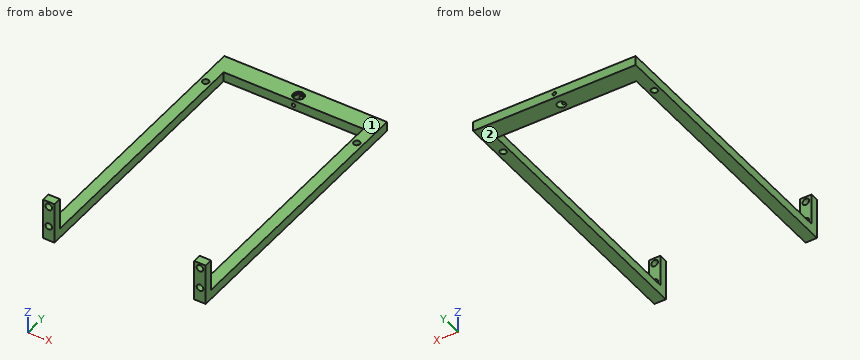
from build123d import *

# Parameters (mm, degrees)
SKETCH1_W           = 99.5426
SKETCH1_H           = 5.842
BOSS_EXTRUDE1_DEPTH = 170.18
SKETCH2_W           = 85.471
SKETCH2_H           = 158.8
CUT_EXTRUDE1_DEPTH  = 232.802638094
SKETCH3_W           = 7.0358
SKETCH3_H           = 5.08
BOSS_EXTRUDE2_DEPTH = 19.304
SKETCH4_R           = 2.032
CUT_EXTRUDE2_DEPTH  = 235.986581553
SKETCH5_R           = 2.54
CUT_EXTRUDE3_DEPTH  = 233.531671991
SKETCH7_R           = 3.302
CUT_EXTRUDE4_DEPTH  = 1.27
SKETCH10_R          = 1.0795
CUT_EXTRUDE7_DEPTH  = 239.583142552
SKETCH11_R          = 1.778
CUT_EXTRUDE8_DEPTH  = 233.531672065
SKETCH9_R           = 1.905
CUT_EXTRUDE6_DEPTH  = 233.531672065


with BuildPart() as part:
    # Sketch1 → Boss-Extrude1 (new body)
    with BuildSketch(Plane(origin=(0, 0, 0), x_dir=(1, 0, 0), z_dir=(0, 1, 0))):
        with Locations((-107.509028278, 53.855595943)):
            Rectangle(SKETCH1_W, SKETCH1_H)
    extrude(amount=BOSS_EXTRUDE1_DEPTH)

    # Sketch2 → Cut-Extrude1 (cut, through all)
    with BuildSketch(Plane.XY.offset(-50.934595943)):
        with Locations((-107.509028278, 79.4)):
            Rectangle(SKETCH2_W, SKETCH2_H)
    extrude(amount=-CUT_EXTRUDE1_DEPTH, mode=Mode.SUBTRACT)

    # Sketch3 → Boss-Extrude2 (add)
    with BuildSketch(Plane.XY.offset(-50.934595943)):
        with Locations((-153.762428278, 2.54)):
            Rectangle(SKETCH3_W, SKETCH3_H)
        with Locations((-61.255628278, 2.54)):
            Rectangle(SKETCH3_W, SKETCH3_H)
    extrude(amount=BOSS_EXTRUDE2_DEPTH)

    # Sketch4 → Cut-Extrude2 (cut, through all)
    with BuildSketch(Plane(origin=(0, 5.08, 0), x_dir=(1, 0, 0), z_dir=(0, 1, 0))):
        with Locations(Location((-153.762428278, 34.932595943, 0), (0, 0, 180))):
            Circle(SKETCH4_R)
        with Locations(Location((-153.762428278, 47.632595943, 0), (0, 0, 180))):
            Circle(SKETCH4_R)
        with Locations(Location((-61.255628278, 34.932595943, 0), (0, 0, 180))):
            Circle(SKETCH4_R)
        with Locations(Location((-61.255628278, 47.632595943, 0), (0, 0, 180))):
            Circle(SKETCH4_R)
    extrude(amount=-CUT_EXTRUDE2_DEPTH, mode=Mode.SUBTRACT)

    # Sketch5 → Cut-Extrude3 (cut, through all)
    with BuildSketch(Plane.XY.offset(-50.934595943)):
        with Locations((-107.509028278, 163.576)):
            Circle(SKETCH5_R)
    extrude(amount=-CUT_EXTRUDE3_DEPTH, mode=Mode.SUBTRACT)

    # Sketch7 → Cut-Extrude4 (cut)
    with BuildSketch(Plane.XY.offset(-50.934595943)):
        with Locations((-107.509028278, 163.576)):
            Circle(SKETCH7_R)
    extrude(amount=-CUT_EXTRUDE4_DEPTH, mode=Mode.SUBTRACT)

    # Sketch10 → Cut-Extrude7 (cut, through all)
    with BuildSketch(Plane(origin=(0, 170.18, 0), x_dir=(1, 0, 0), z_dir=(0, 1, 0))):
        with Locations(Location((-107.509028278, 53.982595943, 0), (0, 0, 270))):
            Circle(SKETCH10_R)
    extrude(amount=-CUT_EXTRUDE7_DEPTH, mode=Mode.SUBTRACT)

    # Sketch11 → Cut-Extrude8 (cut, through all)
    with BuildSketch(Plane.XY.offset(-50.934595943)):
        with Locations((-153.762428278, 147.116)):
            Circle(SKETCH11_R)
        with Locations((-61.255628278, 147.116)):
            Circle(SKETCH11_R)
    extrude(amount=-CUT_EXTRUDE8_DEPTH, mode=Mode.SUBTRACT)

    # Sketch9 → Cut-Extrude6 (cut, through all)
    with BuildSketch(Plane.XY.offset(-50.934595943)):
        with Locations((-153.762428278, 147.37)):
            Circle(SKETCH9_R)
        with Locations((-61.255628278, 147.37)):
            Circle(SKETCH9_R)
    extrude(amount=-CUT_EXTRUDE6_DEPTH, mode=Mode.SUBTRACT)


solid = part.part
Input: part model. Units: mm. Frame: model coordinates. Face numbers are marked on the shaded views. A direction names the side the tool comes from. Give positions to 0.01 mm unless a question says otherwise; leave off trailing zeros. Write each loop counter-clockwise with the first axis right and the second up, starting at its lowest first coordinate (ties: lowest second). Pieces come first, ordered by that corner, then holes. Notation, with made-up numbers: M 0,26 L 49,26 A8 ccw 49,37 Z; hole C -33,39.25 d10. An arc over 180 degrees is marked long. Use one line per item in the form item = value.
1. Cut plane B-B on z = -41. Return loops of the section in (x, y), and give its area (3 significant figures).
Outcome:
outline = M -157.28,0 L -150.24,0 L -150.24,5.08 L -157.28,5.08 Z; M -64.77,0 L -57.74,0 L -57.74,5.08 L -64.77,5.08 Z
area = 71.5 mm²
2. Reachability of the marked faces 1 and 2 from +Z, -Z, +X, -X, +Y, -Y: full face, straight path, thin tool, end or side. Return the list, or none.
Outcome:
face_1 = +Z, +X, -X, +Y
face_2 = -Z, +X, -X, +Y, -Y
3. Cut plane C-C on x = -138. Return loops of the section in (y, z).
Outcome:
outline = M 158.8,-56.78 L 170.18,-56.78 L 170.18,-50.93 L 158.8,-50.93 Z
4. First-contact query: P1, Ø6, axis at x = -107.51, y = 163.58, coming from the +Z side; P2, Ø6.5, axis at x = -124, z = -53, coming from the -Y side; P3, Ø8, axis at x = -107.51, y = 163.58, coming from the +Z side. Flat tips, straight axial feed; report the tip coordinate or a pass-through.
Outcome:
P1 = -52.2
P2 = 158.8
P3 = -50.93
5. Ray query, L1, parallel to X at y = 51, z = -55; L2, parallel to X at y = 147.37, z = -55.25; L3, parallel to Y at x = -99, z = -52.25. Return the intervals inside material, ascending.
Outcome:
L1 = -157.28 to -150.24, -64.77 to -57.74
L2 = -157.28 to -155.67, -151.86 to -150.24, -64.77 to -63.16, -59.35 to -57.74
L3 = 158.8 to 170.18
6. Cut plane A-A on y = 151.5. Return loops of the section in (x, z).
Outcome:
outline = M -157.28,-56.78 L -150.24,-56.78 L -150.24,-50.93 L -157.28,-50.93 Z; M -64.77,-56.78 L -57.74,-56.78 L -57.74,-50.93 L -64.77,-50.93 Z
